from build123d import *

# Parameters (mm, degrees)
SKETCH2_W           = 101.6
SKETCH2_H           = 50.8
SKETCH2_R           = 3.2639
BOSS_EXTRUDE1_DEPTH = 3.175


with BuildPart() as part:
    # Sketch2 → Boss-Extrude1 (new body)
    with BuildSketch(Plane(origin=(0, 0, 0), x_dir=(1, 0, 0), z_dir=(0, 1, 0))):
        with Locations((50.8, 25.4)):
            Rectangle(SKETCH2_W, SKETCH2_H)
        with Locations((50.8, 26.191302461)):
            Circle(SKETCH2_R, mode=Mode.SUBTRACT)
        with BuildLine():
            Line((28.5115, 6.363982324), (28.5115, 46.018622597))
            ThreePointArc((28.5115, 46.018622597), (30.1625, 47.669622597), (31.8135, 46.018622597))
            Line((31.8135, 46.018622597), (31.8135, 6.363982324))
            ThreePointArc((31.8135, 6.363982324), (30.1625, 4.712982324), (28.5115, 6.363982324))
        make_face(mode=Mode.SUBTRACT)
        with BuildLine():
            Line((73.0885, 6.363982324), (73.0885, 46.018622597))
            ThreePointArc((73.0885, 46.018622597), (71.4375, 47.669622597), (69.7865, 46.018622597))
            Line((69.7865, 46.018622597), (69.7865, 6.363982324))
            ThreePointArc((69.7865, 6.363982324), (71.4375, 4.712982324), (73.0885, 6.363982324))
        make_face(mode=Mode.SUBTRACT)
    extrude(amount=BOSS_EXTRUDE1_DEPTH)


solid = part.part
Work out the finished part from the listing and answer in its coordinate system (mm). A direction names the side the tool comes from. Round coordinates to 2 decimals unless told otherwise and drop trailing zeros. Write each loop counter-clockwise with the first axis right and the second up, starting at its lowest first coordinate (ties: lowest second). Pieces come first, ordered by that corner, then holes.
1) A cutting plane is placed at C-C (y = 0.5). Give the vertices of the cut face in (x, z), plus the area to 3 significant figures.
2) A tool of negligible diameter and unlimited length cuts with its end or side. For faces 1 (the flat face through (69.786, 2, -26)), 2 (the flat face through (50, 2, -50.8)), from which of +Z, -Z, +X, -X, +Y, -Y can it reach the whole face along a straight path? Write none if from no direction.
3) A cutting plane is placed at A-A (z = -16). Give the vertices of the cut face in (x, y) (1 decimal), plus the area to 3 significant figures.
4) Straight lines are drawn through the part: line 1 (X direction, y = 0.7, z = -17.5); line 2 (Z direction, x = 50.8, y = 2.2); line 3 (X direction, y = 2.1, z = -5). For each, find the intervals that lie inside material, in ascending order.
5) The mould has two halves that part along X. Classify faces 3 (the flat face through (0, 2, -25)), 4 (the cylindrical face through (71.47, 1.57, -47.67)), 5 (the flat face through (101.6, 2, -25)), 6 (the flat face through (50, 0, -20)): pulls with the +X half, pulls with the -X half, needs draft (parallel to the pull), parting line crosses it, or undercut.
6) A cutting plane is placed at B-B (x = 50.8). Give the vertices of the cut face in (y, z) (3 decimals).
Completed:
1. outline: (0, -50.8) - (101.6, -50.8) - (101.6, 0) - (0, 0) - close; hole (28.51, -46.02) arc R1.65 ccw to (31.81, -46.02) - (31.81, -6.36) arc R1.65 ccw to (28.51, -6.36) - close; hole circle Ø6.53 at (50.8, -26.19); hole (69.79, -46.02) arc R1.65 ccw to (73.09, -46.02) - (73.09, -6.36) arc R1.65 ccw to (69.79, -6.36) - close
1. area: 4,850 mm2
2. face 1: +Y, -Y
2. face 2: -Z, +X, -X, +Y, -Y
3. outline: (0, 0) - (28.5, 0) - (28.5, 3.2) - (0, 3.2) - close; (31.8, 0) - (69.8, 0) - (69.8, 3.2) - (31.8, 3.2) - close; (73.1, 0) - (101.6, 0) - (101.6, 3.2) - (73.1, 3.2) - close
3. area: 302 mm2
4. line 1: x = 0 to 28.51, 31.81 to 69.79, 73.09 to 101.6
4. line 2: z = -50.8 to -29.46, -22.93 to 0
4. line 3: x = 0 to 29.23, 31.09 to 70.51, 72.37 to 101.6
5. face 3: pulls with the -X half
5. face 4: undercut
5. face 5: pulls with the +X half
5. face 6: needs draft
6. outline: (0, -50.8) - (3.175, -50.8) - (3.175, -29.455) - (0, -29.455) - close; (0, -22.927) - (3.175, -22.927) - (3.175, 0) - (0, 0) - close
